```python
from build123d import *

# Parameters (mm, degrees)
SKETCH1_R           = 8.75
BOSS_EXTRUDE1_DEPTH = 1.8
SKETCH2_76_R        = 7.55
SKETCH3_51_R        = 10.2
SKETCH4_W           = 8.6
SKETCH4_H           = 12.41168804
CUT_EXTRUDE1_DEPTH  = 17.660132214


with BuildPart() as part:
    # Sketch1 → Boss-Extrude1 (new body)
    with BuildSketch(Plane(origin=(0, 0, 0), x_dir=(1, 0, 0), z_dir=(0, 1, 0))):
        with Locations(Location((0, 0, 0), (0, 0, 270))):
            Circle(SKETCH1_R)
    extrude(amount=BOSS_EXTRUDE1_DEPTH)

    # Loft1: read off the stored shape, not the designer's step
    # Loft1: loft between two sections, ruled curve by curve
    loft1_from = [
        Edge.make_bspline([(-0.757744305, 1.8, 8.717128172), (16.67651204, 1.8, 10.232616781), (18.192000649, 1.8, -7.201639563), (0.757744305, 1.8, -8.717128172), (-16.67651204, 1.8, -10.232616781), (-18.192000649, 1.8, 7.201639563), (-0.757744305, 1.8, 8.717128172)], [0, 0, 0, 0, 0.5, 0.5, 0.5, 1, 1, 1, 1], 3, [1, 0.333333333, 0.333333333, 1, 0.333333333, 0.333333333, 1]),
    ]
    loft1_to = [
        Edge.make_bspline([(-3.814399501, 6, 10.742921225), (17.671442948, 6, 18.371720228), (25.300241951, 6, -3.114122222), (3.814399501, 6, -10.742921225), (-17.671442948, 6, -18.371720228), (-25.300241951, 6, 3.114122222), (-3.814399501, 6, 10.742921225)], [0, 0, 0, 0, 0.5, 0.5, 0.5, 1, 1, 1, 1], 3, [1, 0.333333333, 0.333333333, 1, 0.333333333, 0.333333333, 1]),
    ]
    loft1 = Solid(Shell([*[Face.make_surface_from_curves(loft1_from[k], loft1_to[k]) for k in range(1)], Face(Wire(loft1_from)), Face(Wire(loft1_to))]))
    add(loft1)

    # Sketch2<76> → Cut-Loft1 section 0
    with BuildSketch(Plane(origin=(0, 1.8, 0), x_dir=(1, 0, 0), z_dir=(0, 1, 0))):
        Circle(SKETCH2_76_R)
    # Sketch3<51> → Cut-Loft1 section 1
    with BuildSketch(Plane(origin=(0, 6, 0), x_dir=(1, 0, 0), z_dir=(0, 1, 0))):
        Circle(SKETCH3_51_R)
    loft(mode=Mode.SUBTRACT)

    # Sketch4 → Cut-Extrude1 (cut, through all)
    with BuildSketch(Plane(origin=(0, 1.8, 0), x_dir=(1, 0, 0), z_dir=(0, 1, 0))):
        Rectangle(SKETCH4_W, SKETCH4_H)
    extrude(amount=-CUT_EXTRUDE1_DEPTH, mode=Mode.SUBTRACT)


solid = part.part
```
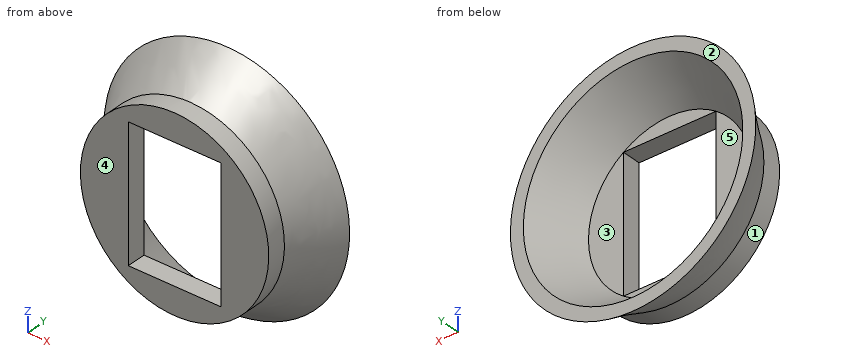
The listing builds one solid part. Answer for the finished solid, in the listing's coordinates (mm). Face numbers are marked on the shaded views. A direction names the side the tool comes from. Give positions to 0.01 mm unless a question says otherwise; leave off trailing zeros. Loops run counter-clockwise (first coordinate to the right, second up) from the corner with the lowest first, then second, coordinate; pieces in that order, holes last. Notation, with made-up numbers: M -8.5,47.25 L 33.5,47.25 A24 cw 33.5,65.25 Z; hole C 22.25,51 d3. An arc over 180 degrees is marked long. One line per item, written item: value.
Q1. For the marked faces 4 and 5, determine the directions among +Z, -Z, +X, -X, +Y, -Y from which every point of the face is accessible in a straight line to the end or side of a thin tool.
Working result:
face 4: +Z, -Z, +X, -X, -Y
face 5: +Y
Q2. Find the intervals of material crossed by line 1 (X direction, y = 3, z = -0.5); line 2 (X direction, y = 0.5, z = -4.5); line 3 (Y direction, x = 6.5, z = -0.75), in increasing order. Write a range as from..to.
Working result:
line 1: x = -9.42..-8.29, 8.29..9.42
line 2: x = -7.5..-4.3, 4.3..7.5
line 3: y = 0..1.8
Q3. A cutting plane is placed at A-A on y = 1. Determine the outline of the cut face in (x, z), then the cut area to 3 significant figures.
Working result:
outline: C 0,0 d17.5; hole M -4.3,-6.21 L 4.3,-6.21 L 4.3,6.21 L -4.3,6.21 Z
area: 134 mm^2
Q4. Determine the mould class of the marked faces 1, 2 and 3 for opening direction Z: +Z half, -Z half, draft (parallel to the pull), parting line (faces both ways), or undercut.
Working result:
face 1: parting line
face 2: draft
face 3: undercut
Q5. Flat-ended cylindrical pins translate along their axes: P1, Ø2, axis at y = 1, z = 2.5, coming from the +X side; P2, Ø0.9, axis at y = 1, z = -2, coming from the -X side; P3, Ø1, axis at x = 5.5, z = -2, coming from the +Y side. Find the tip coordinate at first contact, or state that the pin passes through.
Working result:
P1: stops at x = 8.62
P2: stops at x = -8.61
P3: stops at y = 1.8
